The model under review builds one solid part; all positions refer to its coordinate system, in mm. Give positions to 0.01 mm unless a question says otherwise; leave off trailing zeros. Order: outer loops, then holes, each group sorted by start corner. A loop starts at its lowest first (then second) coordinate and runs counter-clockwise, first axis right, second up. Notation, with made-up numbers: (25, -1.5) - (33, -1.5) arc R10 ccw to (33, 14.5) - close; hole circle Ø6 at (59, 69). An arc over 180 degrees is marked (long way). Put each result on its own line as item: value.
```python
from build123d import *

# Parameters (mm, degrees)
SKETCH1_R           = 15
SKETCH1_R_2         = 1.25
BOSS_EXTRUDE1_DEPTH = 5


with BuildPart() as part:
    # Sketch1 → Boss-Extrude1 (new body)
    with BuildSketch(Plane.XY):
        with BuildLine():
            Line((-33.115304549, -3.323429394), (-5.914945157, -32.079801303))
            ThreePointArc((-5.914945157, -32.079801303), (-1.722792588, -33.954412887), (2.567057485, -32.315663941))
            Line((2.567057485, -32.315663941), (31.323429394, -5.115304549))
            ThreePointArc((31.323429394, -5.115304549), (33.198040978, -0.92315198), (31.559292032, 3.366698093))
            Line((31.559292032, 3.366698093), (4.35893264, 32.123070002))
            ThreePointArc((4.35893264, 32.123070002), (0.166780071, 33.997681586), (-4.123070002, 32.35893264))
            Line((-4.123070002, 32.35893264), (-32.879441911, 5.158573248))
            ThreePointArc((-32.879441911, 5.158573248), (-34.754053495, 0.966420679), (-33.115304549, -3.323429394))
        make_face()
        Circle(SKETCH1_R, mode=Mode.SUBTRACT)
        with Locations((0, 28)):
            Circle(SKETCH1_R_2, mode=Mode.SUBTRACT)
        with Locations((27.200359392, -0.756371909)):
            Circle(SKETCH1_R_2, mode=Mode.SUBTRACT)
        with Locations((-1.556012517, -27.956731301)):
            Circle(SKETCH1_R_2, mode=Mode.SUBTRACT)
        with Locations((-28.756371909, 0.799640608)):
            Circle(SKETCH1_R_2, mode=Mode.SUBTRACT)
    extrude(amount=BOSS_EXTRUDE1_DEPTH)


solid = part.part
```
(1) Take a section at C-C, the plane z = 2.8. Write out the cut boundary in (x, y), then the cut area to 3 significant figures.
The answers:
outline: (-33.12, -3.32) - (-5.91, -32.08) arc R6 ccw to (2.57, -32.32) - (31.32, -5.12) arc R6 ccw to (31.56, 3.37) - (4.36, 32.12) arc R6 ccw to (-4.12, 32.36) - (-32.88, 5.16) arc R6 ccw to start; hole circle Ø2.5 at (-28.76, 0.8); hole circle Ø30 at (0, 0); hole circle Ø2.5 at (-1.56, -27.96); hole circle Ø2.5 at (0, 28); hole circle Ø2.5 at (27.2, -0.76)
area: 1,900 mm^2
(2) Take a section at A-A, the plane y = 28. Write out the cut boundary in (x, z).
The answers:
outline: (-8.73, 0) - (-1.25, 0) - (-1.25, 5) - (-8.73, 5) - close; (1.25, 0) - (8.26, 0) - (8.26, 5) - (1.25, 5) - close
(3) Wall thickness on L1, parallel to Y at x = 0, z = 4.05; L2, parallel to X at y = 12, z = 3.75; L3, parallel to Y at x = 1.5, z = 1.5: over which ranges is each line inside the solid? List them lowest first.
The answers:
L1: -33.75 to -15, 15 to 26.75, 29.25 to 34
L2: -25.65 to -9, 9 to 23.39
L3: -33.12 to -14.92, 14.92 to 33.81
(4) Clearance check with flat-ended pins moving along their axes: pin 1 Ø1.5 at (y, z) = (4, 2) entering from -X; pin 2 Ø1.5 at (x, y) = (0, 28) entering from +Z; pin 3 Ø3 at (x, z) = (-12.5, 3.5) entering from -Y; pin 4 Ø1 at (y, z) = (23.5, 1.5) entering from -X. State where each tip first meets the part, or that it passes through.
The answers:
pin 1: x = -34.23
pin 2: through
pin 3: y = -26.7
pin 4: x = -14.02
(5) The part is to be moulded in two halves that separate along X. For faces 1 (the flat face through (-19.706, -17.5, 2.465)), 2 (the cylindrical face through (-0.27, 26.78, 2.46)), 3 (the cylindrical face through (-14.985, 0.66, 2.465)), 4 (the cylindrical face through (0, 34, 2)), say which applies: pulls with the +X half, pulls with the -X half, needs draft (parallel to the pull), parting line crosses it, or undercut.
The answers:
face 1: pulls with the -X half
face 2: undercut
face 3: undercut
face 4: parting line crosses it
(6) Take a section at D-D, the plane y = -25.5. Write out the cut boundary in (x, z).
The answers:
outline: (-12.14, 0) - (9.77, 0) - (9.77, 5) - (-12.14, 5) - close
(7) Take a section at B-B, the plane x = 12. Write out the cut boundary in (y, z).
The answers:
outline: (-23.39, 0) - (-9, 0) - (-9, 5) - (-23.39, 5) - close; (9, 0) - (24.04, 0) - (24.04, 5) - (9, 5) - close
